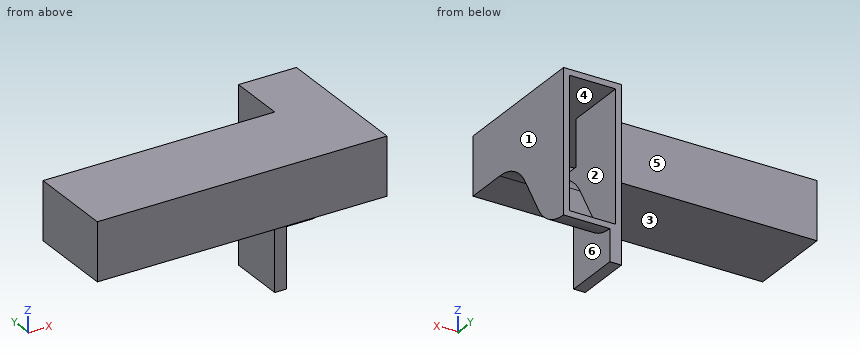
```python
from build123d import *

# Parameters (mm, degrees)
SKETCH1_W           = 40
SKETCH1_H           = 10
BOSS_EXTRUDE1_DEPTH = 15
BOSS_EXTRUDE2_DEPTH = 10
BOSS_EXTRUDE3_DEPTH = 2
SHELL1_START        = -19
SHELL1_OUTLINE_W    = 13
SHELL1_OUTLINE_H    = 8
SHELL1_DEPTH        = 48
SHELL1_START_2      = 21
SHELL1_2_DEPTH      = 8
FILLET1_R           = 4


# Read off the part's stored shape, not the designer's step: Shell1
with BuildPart() as part:
    # Sketch1 → Boss-Extrude1 (new body)
    with BuildSketch(Plane(origin=(0, 0, 0), x_dir=(1, 0, 0), z_dir=(0, 1, 0))):
        with Locations((0, -5)):
            Rectangle(SKETCH1_W, SKETCH1_H)
    extrude(amount=BOSS_EXTRUDE1_DEPTH)

    # Sketch2 → Boss-Extrude2 (add)
    with BuildSketch(Plane(origin=(20, 0, 0), x_dir=(0, 0, -1), z_dir=(1, 0, 0))):
        with BuildLine():
            Line((-10, 0), (-10, 25))
            Line((-10, 25), (14.5, 25))
            ThreePointArc((14.5, 25), (13.42820323, 21), (10.5, 18.07179677))
            Line((10.5, 18.07179677), (4, 14.31902002))
            ThreePointArc((4, 14.31902002), (1.07179677, 11.39081679), (0, 7.39081679))
            Line((0, 7.39081679), (0, 0))
            Line((0, 0), (-10, 0))
        make_face()
    extrude(amount=BOSS_EXTRUDE2_DEPTH)

    # Sketch3 → Boss-Extrude3 (add)
    with BuildSketch(Plane.ZY.offset(-20)):
        with BuildLine():
            Line((-5.179491924, 15), (-20, 15))
            Line((-20, 15), (-20, 25))
            Line((-20, 25), (-14.5, 25))
            ThreePointArc((-14.5, 25), (-13.42820323, 21), (-10.5, 18.07179677))
            Line((-10.5, 18.07179677), (-5.179491924, 15))
        make_face()
    extrude(amount=-BOSS_EXTRUDE3_DEPTH)

    # Shell1 outline → Shell1 (cut)
    with BuildSketch(Plane.YZ.offset(SHELL1_START)):
        with Locations((7.5, 5)):
            Rectangle(SHELL1_OUTLINE_W, SHELL1_OUTLINE_H)
    extrude(amount=SHELL1_DEPTH, mode=Mode.SUBTRACT)

    # Shell1 2 outline → Shell1 2 (cut)
    with BuildSketch(Plane.YZ.offset(SHELL1_START_2)):
        with BuildLine():
            ThreePointArc((18.937822174, -10), (21.5, -12.562177826), (25, -13.5))
            Line((25, -13.5), (25, 9))
            Line((25, 9), (14, 9))
            Line((14, 9), (14, 1))
            Line((14, 1), (7.39081679, 1))
            ThreePointArc((7.39081679, 1), (11.89081679, -0.205771366), (15.185045424, -3.5))
            Line((15.185045424, -3.5), (18.937822174, -10))
        make_face()
    extrude(amount=SHELL1_2_DEPTH, mode=Mode.SUBTRACT)

    # Fillet1
    fillet1_edges = [part.edges().sort_by_distance(p)[0] for p in [
        (-19, 7.5, 1),
        (-19, 7.5, 9),
    ]]
    fillet(fillet1_edges, radius=FILLET1_R - 0.0001)  # a hair under: the kernel refuses the full size


solid = part.part
```
Geometry: final body of the model. Coordinates: model frame, mm. Face numbers are marked on the shaded views. A direction names the side the tool comes from. Coordinates: 2 decimals unless noted, no trailing zeros. Order: outer loops, then holes, each group sorted by start corner. A loop starts at its lowest first (then second) coordinate and runs counter-clockwise, first axis right, second up. Notation, with made-up numbers: (-22.5, -26.75) -> (19.5, -26.75) arc R21 cw to (19.5, 10.25) -> close; hole circle Ø6 at (-16.75, 70). An arc over 180 degrees is marked (long way). Answer in a Markdown table with one row per item.
Item 1: Access query for the marked faces 4, 5 and 6. Directions: +Z, -Z, +X, -X, +Y, -Y. A direction counts if a zero-diameter tool reaches every point of the face in a straight line with its end or side. Return the directions, or none.
Return value:
| item | result |
|---|---|
| face 4 | none |
| face 5 | +Z, -Z, -X, +Y |
| face 6 | -Z, +X, -Y |
Item 2: Section C-C on z = -7.5. Output: boundary loops of the cut face in (x, y).
Return value:
| item | result |
|---|---|
| outline | (20, 15) -> (22, 15) -> (22, 16.34) -> (30, 16.34) -> (30, 25) -> (29, 25) -> (29, 17.49) -> (21, 17.49) -> (21, 25) -> (20, 25) -> close |
Item 3: Section B-B on y = 22.25. Output: boundary loops of the cut face in (x, z), plus the area to 3 significant figures.
Return value:
| item | result |
|---|---|
| outline | (20, -20) -> (22, -20) -> (22, -14.01) -> (30, -14.01) -> (30, 10) -> (20, 10) -> close; hole (21, -12.94) -> (29, -12.94) -> (29, 9) -> (21, 9) -> close |
| area | 76.6 mm² |
Item 4: Ray query, L1, parallel to Z at x = 13.5, y = 7; L2, parallel to Y at x = 1, z = 6.75; L3, parallel to X at y = 10.5, z = 0.5. Return the intervals inside material, ascending.
Return value:
| item | result |
|---|---|
| L1 | z = 0 to 1, 9 to 10 |
| L2 | y = 0 to 1, 14 to 15 |
| L3 | x = -20 to 21, 29 to 30 |
Item 5: Draft query along Z for the marked faces 1, 2 and 3. Return one class per face: released by +Z, released by -Z, zero draft, split by the parting line, or undercut.
Return value:
| item | result |
|---|---|
| face 1 | zero draft |
| face 2 | undercut |
| face 3 | released by -Z |
Item 6: Section A-A on x = -12. Output: boundary loops of the cut face in (y, z), plus the area to 3 significant figures.
Return value:
| item | result |
|---|---|
| outline | (0, 0) -> (15, 0) -> (15, 10) -> (0, 10) -> close; hole (1, 1) -> (14, 1) -> (14, 9) -> (1, 9) -> close |
| area | 46.0 mm² |
Item 7: Contact query for flat-ended pins moving along their axis: P1, Ø8, axis at x = -9, z = 5.5, coming from the +Y side; P2, Ø0.6, axis at x = 21.5, z = -12, coming from the -Y side; P3, Ø12, axis at x = -2, y = 5.5, coming from the -Z side. Output: stop coordinate, or through.
Return value:
| item | result |
|---|---|
| P1 | stops at y = 15 |
| P2 | stops at y = 15 |
| P3 | stops at z = 0 |
